Check sheet for the modelled part. Datum: model origin and axes. Units: mm. Face numbers are marked on the shaded views. A direction names the side the tool comes from. Give positions to 0.01 mm unless a question says otherwise; leave off trailing zeros. Order: outer loops, then holes, each group sorted by start corner. A loop starts at its lowest first (then second) coordinate and runs counter-clockwise, first axis right, second up. Notation, with made-up numbers: (34.25, -37) -> (80.25, -37) arc R13 ccw to (80.25, -32) -> close; hole circle Ø4 at (44, 79.25). An arc over 180 degrees is marked (long way). Answer in a Markdown table with one row per item. Add a question column.
(1) Thickness scan on L1, parallel to X at y = 12.5, z = 8; L2, parallel to Z at x = 33.5, y = 1.2; L3, parallel to Z at x = 33.5, y = 0.95. Record the ranges inside material, lowest first. Write a range as [from, to].
(2) Set-up check for the marked faces 5, 6 and 7: record each of +Z, -Z, +X, -X, +Y, -Y from which the full face is reachable in a straight line by a thin tool's end or side.
(3) Cross-section at A-A (x = 33.5). Record the cut outline in (y, z), then the cut area to 3 significant figures.
(4) Cross-section at B-B (y = 40). Record the cut outline in (x, z), then the cut area to 3 significant figures.
(5) Release check for a two-part mould opening along X. For the marked faces 1, 2, 3 and 4 record: released by +X, released by -X, zero draft, split by the parting line, or undercut.
(6) Cross-section at C-C (z = 0). Record the cut outline in (x, y), then the cut area to 3 significant figures.
(7) Cross-section at D-D (z = -18.5). Record the cut outline in (x, y), then the cut area to 3 significant figures.
(8) Go/stop test with flat-tipped pins: pin 1 (10 mm diameter, centred on x = 42.5, z = 1.5, fed in from +Y); pin 2 (3.5 mm diameter, centred on x = 33.5, z = 16.9, fed in from -Y). Record where each tip stops, or that it passes through.
Autodesk Inventor part; units mm, degrees
ref_plane "Work Plane1" through (0, 2, -22.5) normal (0, -1, 0) x (1, 0, 0)
ref_plane "YZ Plane" through (0, 0, 0) normal (1, 0, 0) x (0, 1, 0)
ref_plane "XZ Plane" through (0, 0, 0) normal (0, 1, 0) x (-1, 0, 0)
sketch "Sketch1" plane through (0, 0, 0) normal (1, 0, 0) x (0, 1, 0)
  circle A0 centre (40, 0) radius 32 construction
  arc A1 (42.8857, -9.5746) -> (42.8857, 9.5746) centre (40, 0) ccw
  line L0 (42.8857, -9.5746) -> (0, -22.5)
  line L1 (0, -22.5) -> (0, 0)
  line L2 (0, 0) -> (28, 0) construction
  line L3 (42.8857, 9.5746) -> (0, 22.5)
  line L4 (0, 22.5) -> (0, 0)
  line L5 (40, 0) -> (28, 0) construction
  dimension "d0" = 20
  dimension "d1" = 64
  dimension "d2" = 40
  dimension "d3" = 45
extrude "Extrusion1" add sketch "Sketch1" along normal blind 67
ref_plane "Work Plane1" through (0, 2, -22.5) normal (0, -1, 0) x (1, 0, 0)
sketch "Sketch2" plane through (0, 2, -22.5) normal (0, -1, 0) x (1, 0, 0)
  line L0 (0, 45) -> (0, 0) construction
  line L1 (0, 0) -> (67, 0) construction
  line L2 (67, 45) -> (67, 0) construction
  line L3 (0, 45) -> (67, 45) construction
  line L4 (0, 45) -> (67, 45) construction
  line L5 (0, 0) -> (67, 0) construction
  line L6 (64, 45) -> (3, 45)
  line L7 (3, 45) -> (3, 0)
  line L8 (3, 0) -> (64, 0)
  line L9 (64, 0) -> (64, 45)
  line L10 (67, 45) -> (67, 0)
  line L11 (67, 22.5) -> (64, 22.5) construction
  line L12 (0, 22.5) -> (3, 22.5) construction
  dimension "d7" = 61
extrude "Extrusion2" cut sketch "Sketch2" against normal through all
sketch "Sketch3" plane through (3, 2, 21.8972) normal (1, 0, 0) x (0, 0, -1)
  arc A0 (31.4718, 40.8857) -> (12.3226, 40.8857) centre (21.8972, 38) ccw
  circle A1 centre (21.8972, 38) radius 10
  point P0 (21.8972, -2)
extrude "Extrusion3" add sketch "Sketch3" along normal blind 3
sketch "Sketch4" plane through (64, 2, -21.8972) normal (-1, 0, 0) x (0, 0, 1)
  arc A0 (31.4718, 40.8857) -> (12.3226, 40.8857) centre (21.8972, 38) ccw
  circle A1 centre (21.8972, 38) radius 10
  point P0 (21.8972, -2)
  point P1 (12.3226, 40.8857)
extrude "Extrusion4" add sketch "Sketch4" along normal blind 3
fillet "Fillet1" radius 4 2 edges at (64, 2, 0) (3, 2, 0)
sketch "Sketch5" plane through (0, 2, -22.5) normal (0, 1, 0) x (1, 0, 0)
  line L0 (60, -44.3972) -> (7, -44.3972)
  line L1 (33.5, -44.3972) -> (33.5, -0.6028) construction
  line L2 (7, -0.6028) -> (60, -0.6028)
  circle A0 centre (33.5, -39.3972) radius 2.75
  circle A1 centre (33.5, -5.6028) radius 2.75
  point P0 (0, -22.5)
  dimension "d18" = 5
  dimension "d19" = 5.5
  dimension "d20" = 5
extrude "Extrusion5" cut sketch "Sketch5" against normal blind 3
properties part number "SpoolHolder"
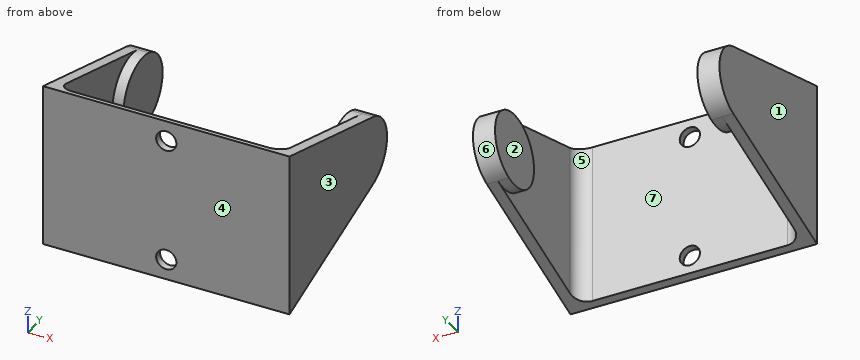
Answer below:
| question | item | result |
|---|---|---|
| 1 | L1 | x = [0, 3], [64, 67] |
| 1 | L2 | z = [-22.14, -19.65], [-14.15, 14.15], [19.65, 22.14] |
| 1 | L3 | z = [-22.21, -19.65], [-14.15, 14.15], [19.65, 22.21] |
| 2 | face 5 | +Z, -Z |
| 2 | face 6 | +X, -X, +Y |
| 2 | face 7 | +Z, -Z, +Y |
| 3 | outline | (0, -22.5) -> (2, -21.9) -> (2, -19.65) -> (0, -19.65) -> close; (0, -14.15) -> (2, -14.15) -> (2, 14.15) -> (0, 14.15) -> close; (0, 19.65) -> (2, 19.65) -> (2, 21.9) -> (0, 22.5) -> close |
| 3 | area | 66.8 mm² |
| 4 | outline | (0, -10.44) -> (3, -10.44) -> (3, -10) -> (6, -10) -> (6, 10) -> (3, 10) -> (3, 10.44) -> (0, 10.44) -> close; (61, -10) -> (64, -10) -> (64, -10.44) -> (67, -10.44) -> (67, 10.44) -> (64, 10.44) -> (64, 10) -> (61, 10) -> close |
| 4 | area | 245 mm² |
| 5 | face 1 | released by -X |
| 5 | face 2 | undercut |
| 5 | face 3 | released by +X |
| 5 | face 4 | zero draft |
| 6 | outline | (0, 0) -> (67, 0) -> (67, 50) -> (61, 50) -> (61, 30) -> (64, 30) -> (64, 6) arc R4 cw to (60, 2) -> (7, 2) arc R4 cw to (3, 6) -> (3, 30) -> (6, 30) -> (6, 50) -> (0, 50) -> close |
| 6 | area | 549 mm² |
| 7 | outline | (0, 0) -> (31.27, 0) -> (31.27, 2) -> (7, 2) arc R4 cw to (3, 6) -> (3, 13.27) -> (0, 13.27) -> close; (35.73, 0) -> (67, 0) -> (67, 13.27) -> (64, 13.27) -> (64, 6) arc R4 cw to (60, 2) -> (35.73, 2) -> close |
| 7 | area | 200 mm² |
| 8 | pin 1 | stops at y = 2 |
| 8 | pin 2 | passes through |
